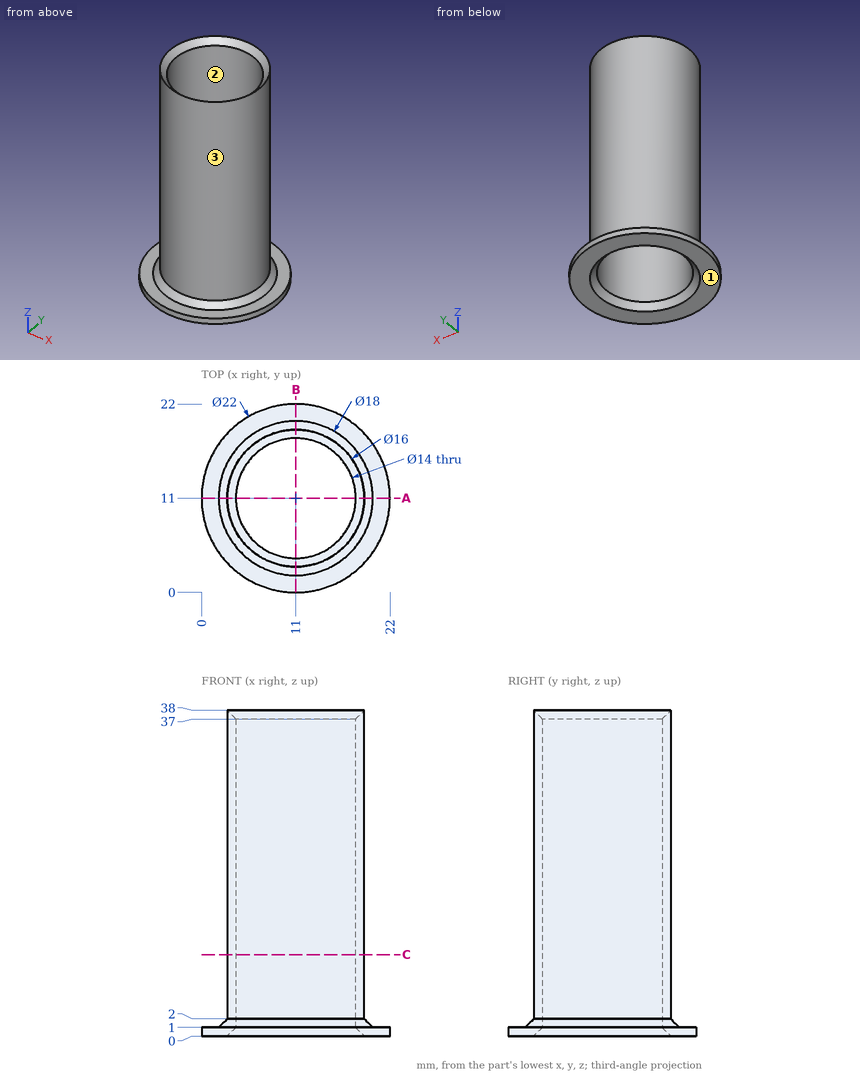
Job drawing, mm, ordinate dimensions from the low corner. One solid piece. Give positions to 0.01 mm unless a question says otherwise; leave off trailing zeros. Order: outer loops, then holes, each group sorted by start corner. A loop starts at its lowest first (then second) coordinate and runs counter-clockwise, first axis right, second up. Notation, with made-up numbers: M -15,75 L 15,75 A33 ccw 15,104 Z; hole C -29.5,-32.5 d3. An arc over 180 degrees is marked long. Put each result on its own line as item: value. Start each with the question number.
(1) Drill centre lines: L1, parallel to Y at x = 11, z = 21; L2, parallel to Y at x = 17, z = 10; L3, parallel to X at y = 8, z = 28. Where is each one in solid material? Low to high. Write a range as [from, to].
(2) Band-saw the part on A-A on y = 11. Give the cut face in (x, z), then the cut area to 3 significant figures.
(3) Pull direction Y, two halves, no side cores. Call the marked faces 1, 2 and 3: released by +Y, released by -Y, zero draft, split by the parting line, or undercut.
(4) Pin check, flat tips, straight feed: pin 1 Ø3 at (y, z) = (16, 5.5) entering from +X; pin 2 Ø3 at (x, y) = (19.5, 3) entering from +Z; pin 3 Ø8 at (x, z) = (19, 21) entering from +Y. Stop position of each tip, or through.
(5) Band-saw the part on C-C on z = 9.5. Give the cut face in (x, y).
Results below:
1. L1: y = [3, 4], [18, 19]
1. L2: y = [5.71, 7.39], [14.61, 16.29]
1. L3: x = [3.58, 4.68], [17.32, 18.42]
2. outline: M 0,0 L 3,0 L 4,1 L 4,37 L 3,38 L 3,2 L 2,1 L 0,1 Z; M 18,1 L 19,0 L 22,0 L 22,1 L 20,1 L 19,2 L 19,38 L 18,37 Z
2. area: 81.0 mm2
3. face 1: zero draft
3. face 2: undercut
3. face 3: split by the parting line
4. pin 1: stops at x = 18.19
4. pin 2: stops at z = 1
4. pin 3: stops at y = 17.93
5. outline: C 11,11 d16; hole C 11,11 d14
